Can you work these out from the model? Positions are in its coordinate system, mm. Round coordinates to 2 decimals unless told otherwise and drop trailing zeros. Loops run counter-clockwise (first coordinate to the right, second up) from the corner with the lowest first, then second, coordinate; pieces in that order, holes last. Notation, with made-up numbers: (32.25, 32.25) -> (82.25, 32.25) arc R4 cw to (82.25, 37.25) -> close; hole circle Ø10 at (55, -37). An arc over 180 degrees is marked (long way). Answer as a JSON object with one key per item and string values.
Autodesk Inventor part; units mm, degrees
ref_plane "YZ Plane" through (0, 0, 0) normal (1, 0, 0) x (0, 1, 0)
ref_plane "XZ Plane" through (0, 0, 0) normal (0, 1, 0) x (-1, 0, 0)
ref_plane "XY Plane" through (0, 0, 0) normal (0, 0, 1) x (1, 0, 0)
sketch "Sketch1" plane through (0, 0, 0) normal (0, 0, 1) x (1, 0, 0)
  line L0 (-35.3228, 16.049) -> (-9.9228, 16.049)
  line L1 (-9.9228, 16.049) -> (-9.9228, -34.751)
  line L2 (-9.9228, -34.751) -> (-35.3228, -34.751)
  line L3 (-35.3228, -34.751) -> (-35.3228, 16.049)
  line L4 (-13.0978, 12.874) -> (-32.1478, 12.874)
  line L5 (-32.1478, 12.874) -> (-32.1478, -31.576)
  line L6 (-32.1478, -31.576) -> (-13.0978, -31.576)
  line L7 (-13.0978, -31.576) -> (-13.0978, 12.874)
  point P0 (0, 0)
  dimension "d0" = 25.4
  dimension "d1" = 50.8
  dimension "d2" = 3.175
extrude "Extrusion1" add sketch "Sketch1" along normal blind 977.9
sketch "Sketch2" plane through (-35.3228, -34.751, 0) normal (-1, 0, 0) x (0, 0, 1)
  line L0 (0, 0) -> (0, 50.8) construction
  line L1 (0, 25.4) -> (25.4, 25.4) construction
  circle A0 centre (25.4, 25.4) radius 14.2875
  point P0 (0, 34.751)
  dimension "d5" = 25.4
  dimension "d9" = 28.575
extrude "Extrusion2" cut sketch "Sketch2" against normal blind 12.7
sketch "Sketch3" plane through (-35.3228, -34.751, 0) normal (-1, 0, 0) x (0, 0, 1)
  line L0 (977.9, 50.8) -> (977.9, 0) construction
  line L1 (977.9, 25.4) -> (800.1, 25.4) construction
  circle A0 centre (800.1, 25.4) radius 14.2875
  point P0 (0, 34.751)
  dimension "d10" = 177.8
  dimension "d11" = 28.575
extrude "Extrusion3" cut sketch "Sketch3" against normal blind 25.4
sketch "Sketch7" plane through (-9.9228, -34.751, 0) normal (1, 0, 0) x (0, 0, -1)
  line L0 (0, 0) -> (0, 50.8) construction
  line L1 (0, 25.4) -> (-25.4, 25.4) construction
  circle A0 centre (-25.4, 25.4) radius 12.7
  point P0 (0, 34.751)
  dimension "d34" = 25.4
  dimension "d35" = 25.4
extrude "Extrusion7" cut sketch "Sketch7" against normal blind 12.7
sketch "Sketch9" plane through (-9.9228, -34.751, 0) normal (1, 0, 0) x (0, 0, -1)
  circle A0 centre (-25.4, 25.4) radius 12.7 construction
  line L0 (-25.4, 25.4) -> (-25.4, 49.2125) construction
  line L1 (-25.4, 49.2125) -> (-4.7778, 37.3063) construction
  line L2 (-4.7778, 37.3063) -> (-4.7778, 13.4938) construction
  line L3 (-4.7778, 13.4938) -> (-25.4, 1.5875) construction
  line L4 (-25.4, 1.5875) -> (-46.0222, 13.4937) construction
  line L5 (-46.0222, 13.4937) -> (-46.0222, 37.3062) construction
  line L6 (-46.0222, 37.3062) -> (-25.4, 49.2125) construction
  circle A1 centre (-4.7778, 37.3063) radius 2.5797
  circle A2 centre (-4.7778, 13.4938) radius 2.5797
  circle A3 centre (-46.0222, 13.4938) radius 2.5797
  circle A4 centre (-46.0222, 37.3062) radius 2.5797
  point P0 (0, 34.751)
  dimension "d44" = 23.8125
  dimension "d45" = 5.1594
  dimension "d46" = 5.1594
  dimension "d47" = 5.1594
  dimension "d48" = 5.1594
extrude "Extrusion9" cut sketch "Sketch9" against normal blind 25.4
sketch "Sketch10" plane through (0, 0, 0) normal (0, 0, -1) x (-1, 0, 0)
  line L0 (35.3228, 16.049) -> (9.9228, 16.049)
  line L1 (9.9228, 16.049) -> (13.0978, 16.049)
  line L2 (13.0978, 16.049) -> (13.0978, -34.751)
  line L3 (13.0978, -34.751) -> (9.9228, -34.751)
  line L4 (9.9228, -34.751) -> (9.9228, 16.049)
  line L5 (9.9228, -34.751) -> (35.3228, -34.751)
  line L6 (9.9228, -34.751) -> (35.3228, -34.751)
  line L7 (35.3228, -34.751) -> (35.3228, -31.576)
  line L8 (35.3228, -31.576) -> (9.9228, -31.576)
  line L9 (9.9228, -31.576) -> (9.9228, -34.751)
  line L10 (35.3228, -34.751) -> (32.1478, -34.751)
  line L11 (32.1478, -34.751) -> (32.1478, 16.049)
  line L12 (32.1478, 16.049) -> (35.3228, 16.049)
  line L13 (35.3228, 16.049) -> (35.3228, -34.751)
  line L14 (9.9228, 16.049) -> (35.3228, 16.049)
  line L15 (35.3228, 16.049) -> (35.3228, 12.874)
  line L16 (35.3228, 12.874) -> (9.9228, 12.874)
  line L17 (9.9228, 12.874) -> (9.9228, 16.049)
  point P0 (0, 0)
  dimension "d51" = 3.175
  dimension "d52" = 50.8
  dimension "d53" = 25.4
  dimension "d54" = 3.175
  dimension "d55" = 3.175
  dimension "d56" = 50.8
  dimension "d57" = 25.4
  dimension "d58" = 3.175
extrude "Extrusion10" add sketch "Sketch10" along normal blind 12.7 contours L13 L16 L11 L0 | L11 L16 L2 L0 | L13 L8 L11 L16 | L2 L16 L4 L0 | L7 L5 L11 L8 | L2 L8 L4 L16 | L11 L5 L2 L8 | L2 L3 L4 L8
properties part number "41.75in Arm Beam Alternate (Left)"
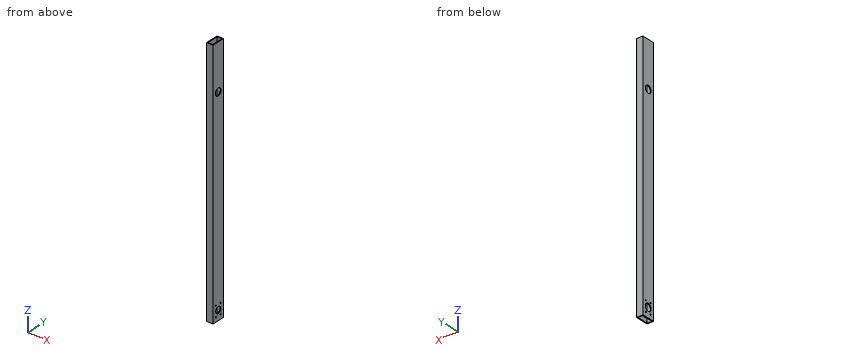
Q1. I'm going to push a flat-ended pin straight in: pin 1 (8 mm diameter, centred on x = -32, y = 9.5, fed in from +Z). Where does the tip first touch, or does it pass through?
Determined:
{"pin 1": "z = 977.9"}
Q2. I want a section at A-A, the plane z = 800.1. Write out the boundary of the cut face in (x, y).
Determined:
{"outline": "(-35.32, -34.75) -> (-9.92, -34.75) -> (-9.92, -23.64) -> (-13.1, -23.64) -> (-13.1, -31.58) -> (-32.15, -31.58) -> (-32.15, -23.64) -> (-35.32, -23.64) -> close; (-35.32, 4.94) -> (-32.15, 4.94) -> (-32.15, 12.87) -> (-13.1, 12.87) -> (-13.1, 4.94) -> (-9.92, 4.94) -> (-9.92, 16.05) -> (-35.32, 16.05) -> close"}
Q3. I want a section at D-D, the plane z = 25.4. Write out the boundary of the cut face in (x, y), then the cut area to 3 significant figures.
Determined:
{"outline": "(-35.32, -34.75) -> (-9.92, -34.75) -> (-9.92, -22.05) -> (-13.1, -22.05) -> (-13.1, -31.58) -> (-32.15, -31.58) -> (-32.15, -23.64) -> (-35.32, -23.64) -> close; (-35.32, 4.94) -> (-32.15, 4.94) -> (-32.15, 12.87) -> (-13.1, 12.87) -> (-13.1, 3.35) -> (-9.92, 3.35) -> (-9.92, 16.05) -> (-35.32, 16.05) -> close", "area": "272 mm²"}
Q4. I want a section at C-C, the plane z = 251.5. Write out the boundary of the cut face in (x, y).
Determined:
{"outline": "(-35.32, -34.75) -> (-9.92, -34.75) -> (-9.92, 16.05) -> (-35.32, 16.05) -> close; hole (-32.15, -31.58) -> (-13.1, -31.58) -> (-13.1, 12.87) -> (-32.15, 12.87) -> close"}
Q5. If I drill on L1, parallel to X at y = -8, z = 769; L2, parallel to Y at x = -18, z = 436.5; L3, parallel to Y at x = -12, z = 800.1, over which ranges is the centre line in solid material (lowest first)? Write a range as [from, to].
Determined:
{"L1": "[-35.32, -32.15], [-13.1, -9.92]", "L2": "[-34.75, -31.58], [12.87, 16.05]", "L3": "[-34.75, -23.64], [4.94, 16.05]"}
Q6. I want a section at B-B, the plane x = -26.25. Write out the boundary of the cut face in (y, z), then the cut area to 3 significant figures.
Determined:
{"outline": "(-34.75, -12.7) -> (-31.58, -12.7) -> (-31.58, 977.9) -> (-34.75, 977.9) -> close; (12.87, -12.7) -> (16.05, -12.7) -> (16.05, 977.9) -> (12.87, 977.9) -> close", "area": "6,290 mm²"}
